from build123d import *

# Parameters (mm, degrees)
SKETCH_1_W          = 116
SKETCH_1_H          = 84.18
SKETCH_1_R          = 1.5
EXTRUDE_1_DEPTH     = 3
CUT_EXTRUDE_1_DEPTH = 10
EXTRUDE_2_DEPTH     = 3
SKETCH_10_R         = 1.5
CUT_EXTRUDE_2_DEPTH = 149.309542849
CUT_EXTRUDE_3_DEPTH = 149.309542849
FILLET_2_R          = 2
FILLET_3_R          = 2
SKETCH_12_R         = 1.5
CUT_EXTRUDE_4_DEPTH = 10


with BuildPart() as part:
    # 草图1 → 凸台-拉伸1 (new body)
    with BuildSketch(Plane(origin=(0, 0, 0), x_dir=(1, 0, 0), z_dir=(0, 1, 0))):
        Rectangle(SKETCH_1_W, SKETCH_1_H)
        with Locations(Location((-40, 36.09, 0), (0, 0, 270))):
            Circle(SKETCH_1_R, mode=Mode.SUBTRACT)
        with Locations(Location((-20, 36.09, 0), (0, 0, 270))):
            Circle(SKETCH_1_R, mode=Mode.SUBTRACT)
        with Locations(Location((-48.125, 16.09, 0), (0, 0, 270))):
            Circle(SKETCH_1_R, mode=Mode.SUBTRACT)
        with Locations(Location((-48.125, -3.91, 0), (0, 0, 270))):
            Circle(SKETCH_1_R, mode=Mode.SUBTRACT)
        with Locations(Location((48.125, -3.91, 0), (0, 0, 90))):
            Circle(SKETCH_1_R, mode=Mode.SUBTRACT)
        with Locations(Location((48.125, 16.09, 0), (0, 0, 90))):
            Circle(SKETCH_1_R, mode=Mode.SUBTRACT)
        with Locations(Location((20, 36.09, 0), (0, 0, 90))):
            Circle(SKETCH_1_R, mode=Mode.SUBTRACT)
        with Locations(Location((40, 36.09, 0), (0, 0, 90))):
            Circle(SKETCH_1_R, mode=Mode.SUBTRACT)
        with Locations(Location((40, -36.09, 0), (0, 0, 270))):
            Circle(SKETCH_1_R, mode=Mode.SUBTRACT)
        with Locations(Location((20, -36.09, 0), (0, 0, 270))):
            Circle(SKETCH_1_R, mode=Mode.SUBTRACT)
        with Locations(Location((-20, -36.09, 0), (0, 0, 90))):
            Circle(SKETCH_1_R, mode=Mode.SUBTRACT)
        with Locations(Location((-40, -36.09, 0), (0, 0, 90))):
            Circle(SKETCH_1_R, mode=Mode.SUBTRACT)
    extrude(amount=EXTRUDE_1_DEPTH)

    # 草图2 → 切除-拉伸1 (cut)
    with BuildSketch(Plane(origin=(0, 3, 0), x_dir=(1, 0, 0), z_dir=(0, 1, 0))):
        with BuildLine():
            Line((-25, 20), (25, 20))
            ThreePointArc((25, 20), (32.5, 12.5), (25, 5))
            Line((25, 5), (-25, 5))
            ThreePointArc((-25, 5), (-32.5, 12.5), (-25, 20))
        make_face()
        with BuildLine():
            Line((-25, -20), (25, -20))
            ThreePointArc((25, -20), (32.5, -12.5), (25, -5))
            Line((25, -5), (-25, -5))
            ThreePointArc((-25, -5), (-32.5, -12.5), (-25, -20))
        make_face()
    extrude(amount=-CUT_EXTRUDE_1_DEPTH, mode=Mode.SUBTRACT)

    # 草图4 → 凸台-拉伸2 (add)
    with BuildSketch(Plane(origin=(0, 3, 0), x_dir=(1, 0, 0), z_dir=(0, 1, 0))):
        Polygon((58, 42.09), (142.18, 42.09), (58, -42.09), align=None)
        Polygon((-58, -42.09), (-58, 42.09), (-142.18, 42.09), align=None)
    extrude(amount=-EXTRUDE_2_DEPTH)

    # 草图10 → 切除-拉伸2 (cut, through all)
    with BuildSketch(Plane(origin=(0, 0, 0), x_dir=(-1, 0, 0), z_dir=(0, -1, 0))):
        with Locations(Location((69.000844337, -23.24902983, 0), (0, 0, 90))):
            Circle(SKETCH_10_R)
        with Locations(Location((83.142979961, -9.106894206, 0), (0, 0, 90))):
            Circle(SKETCH_10_R)
        with Locations(Location((-83.142979961, -9.106894206, 0), (0, 0, 270))):
            Circle(SKETCH_10_R)
        with Locations(Location((-69.000844337, -23.24902983, 0), (0, 0, 270))):
            Circle(SKETCH_10_R)
    extrude(amount=-CUT_EXTRUDE_2_DEPTH, mode=Mode.SUBTRACT)

    # 草图11 → 切除-拉伸3 (cut, through all)
    with BuildSketch(Plane(origin=(0, 3, 0), x_dir=(1, 0, 0), z_dir=(0, 1, 0))):
        Polygon((-105.197738543, 27.09), (-58.125, 27.09), (-58.125, -19.982738543), align=None)
        Polygon((58.125, -19.982738543), (105.197738543, 27.09), (58.125, 27.09), align=None)
    extrude(amount=-CUT_EXTRUDE_3_DEPTH, mode=Mode.SUBTRACT)

    # 圆角2
    fillet_2_edges = [part.edges().sort_by_distance(p)[0] for p in [
        (-58.125, 1.5, 19.982738543),
        (-105.197738543, 1.5, -27.09),
        (-58.125, 1.5, -27.09),
        (58.125, 1.5, 19.982738543),
        (58.125, 1.5, -27.09),
        (105.197738543, 1.5, -27.09),
    ]]
    fillet(fillet_2_edges, radius=FILLET_2_R)

    # 圆角3
    fillet_3_edges = [part.edges().sort_by_distance(p)[0] for p in [
        (142.18, 1.5, -42.09),
        (-142.18, 1.5, -42.09),
        (58, 1.5, 42.09),
        (-58, 1.5, 42.09),
    ]]
    fillet(fillet_3_edges, radius=FILLET_3_R)

    # 草图12 → 切除-拉伸4 (cut)
    with BuildSketch(Plane(origin=(0, 0, 0), x_dir=(-1, 0, 0), z_dir=(0, -1, 0))):
        with Locations(Location((-100, 36.089415022, 0), (0, 0, 90))):
            Circle(SKETCH_12_R)
        with Locations(Location((-80, 36.089415022, 0), (0, 0, 90))):
            Circle(SKETCH_12_R)
        with Locations(Location((80, 36.089415022, 0), (0, 0, 270))):
            Circle(SKETCH_12_R)
        with Locations(Location((100, 36.089415022, 0), (0, 0, 270))):
            Circle(SKETCH_12_R)
    extrude(amount=-CUT_EXTRUDE_4_DEPTH, mode=Mode.SUBTRACT)


solid = part.part
Read the model definition and answer for the solid it produces. Units are mm, in the model's axes. A direction names the side the tool comes from. Coordinates: 2 decimals unless noted, no trailing zeros. Loops run counter-clockwise (first coordinate to the right, second up) from the corner with the lowest first, then second, coordinate; pieces in that order, holes last. Notation, with made-up numbers: (59, 5.5) -> (102, 5.5) arc R18 ccw to (102, 22.5) -> close; hole circle Ø7 at (38.25, -23.75). An arc over 180 degrees is marked (long way). Write item = value, one per line. Start each with the question number.
1) The part is cut by section A-A, the plane z = -1.5. Determine the outline of the cut face in (x, y) (3 decimals).
2) Find the intervals of material crossed by L1, parallel to Z at x = 2, y = 1.25; L2, parallel to Z at x = 48, y = 1.2; L3, parallel to X at y = 1.4, z = -26.5, in increasing order. Write a range as from..to.
3) Given P1, Ø1.8, axis at x = 40, z = 36.09, coming from the +Y side, flat-ended and moving along its own axis, determine where the tip first touches the part or whether it passes through.
4) The mould has two halves that part along Z. Classify faces 1 (the face through (2, 3, -1)), 2 (the face through (99.24, 1.52, 0.85)), 3 (the face through (32.5, 1.52, -12.66)), 4 (the face through (-81.38, 1.52, -3.27)): pulls with the +Z half, pulls with the -Z half, needs draft (parallel to the pull), parting line crosses it, or undercut.
5) The part is cut by section B-B, the plane x = -120.5. Determine the outline of the cut face in (y, z).
6) The part is cut by section D-D, the plane x = 122.5. Determine the outline of the cut face in (y, z).
7) For faces 5 (the face through (-32.5, 1.52, -12.34)), 6 (the face through (-99.24, 1.52, 0.85)), determine the directions among +Z, -Z, +X, -X, +Y, -Y from which every point of the face is accessible in a straight line to the end or side of a thin tool.
8) The part is cut by section C-C, the plane y = 0.65. State how many separate pieces and enclosed holes the cut face has, plus the area to 3 significant figures.
Result:
q1.outline = (-101.59, 0) -> (-79.608, 0) -> (-79.608, 3) -> (-101.59, 3) -> close; (-58.125, 0) -> (58.125, 0) -> (58.125, 3) -> (-58.125, 3) -> close; (79.608, 0) -> (101.59, 0) -> (101.59, 3) -> (79.608, 3) -> close
q2.L1 = -42.09..-20, -5..5, 20..42.09
q2.L2 = -42.09..-17.58, -14.6..2.42, 5.4..42.09
q2.L3 = -126.59..-101.79, -58.71..58.71, 101.79..126.59
q3.P1 = through
q4.face_1 = needs draft
q4.face_2 = pulls with the +Z half
q4.face_3 = undercut
q4.face_4 = undercut
q5.outline = (0, -42.09) -> (3, -42.09) -> (3, -20.41) -> (0, -20.41) -> close
q6.outline = (0, -42.09) -> (3, -42.09) -> (3, -22.41) -> (0, -22.41) -> close
q7.face_5 = +Y, -Y
q7.face_6 = +Z, -X, +Y, -Y
q8.separate_pieces = 1
q8.enclosed_holes = 24
q8.area = 12,700 mm²
